Could you check a few things on this drawing? It's one solid part, dimensions in mm from its lowest x, y, z. A direction names the side the tool comes from. Give positions to 0.01 mm unless a question says otherwise; leave off trailing zeros. Write each loop counter-clockwise with the first axis right and the second up, starting at its lowest first coordinate (ties: lowest second). Pieces come first, ordered by that corner, then holes. Notation, with made-up numbers: M 50.25,78 L 96.25,78 A31 ccw 96.25,117 Z; hole C 79.25,9.5 d11. An arc over 180 degrees is marked long. Write each question's results on one line, items separated by ' | '.
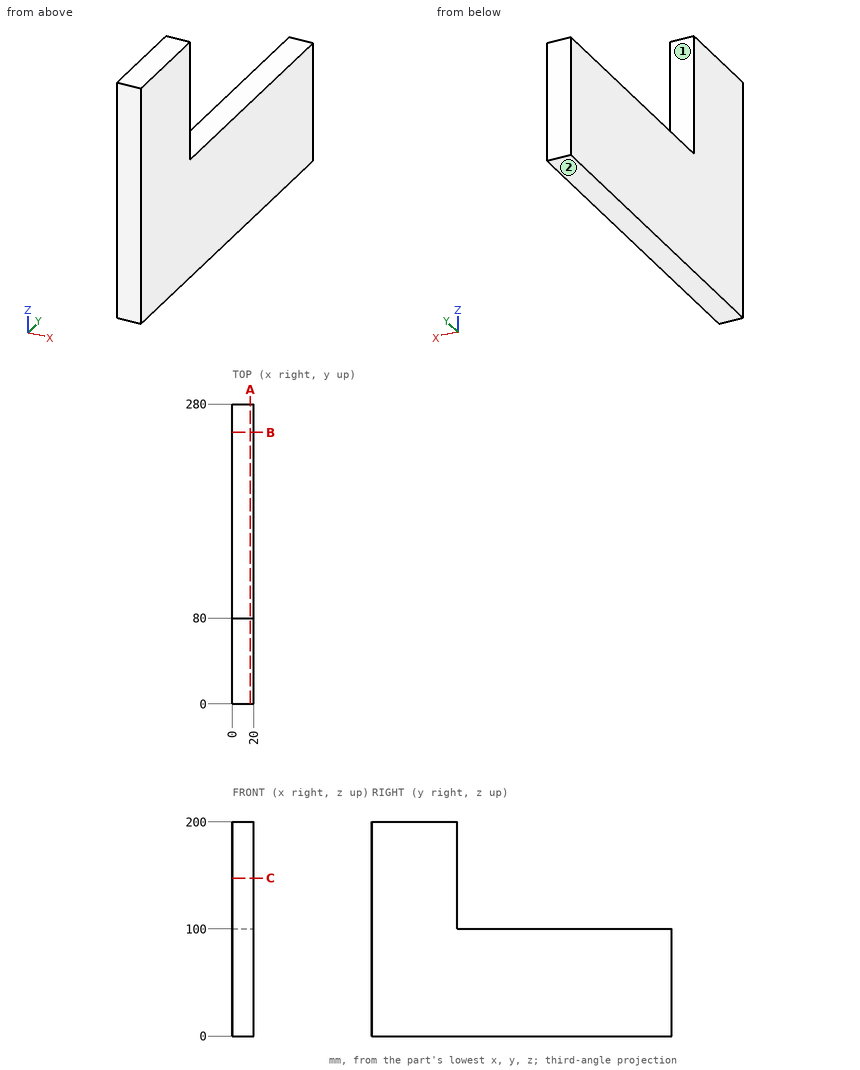
Item 1: I want a section at C-C, the plane z = 147.5. Please give me the cut outline in (x, y).
Geometry says:
outline: M 0,0 L 20,0 L 20,80 L 0,80 Z
Item 2: I want a section at A-A, the plane x = 16.75. Please give me the cut outline in (y, z), and give its area (3 significant figures).
Geometry says:
outline: M 0,0 L 280,0 L 280,100 L 80,100 L 80,200 L 0,200 Z | area: 36,000 mm2
Item 3: I'm going to push flat-ended pins straight in: pin 1 (10 mm diameter, centred on x = 8, z = 157, fed in from +Y); pin 2 (5 mm diameter, centred on x = 10.5, y = 183, fed in from +Z). Where does each tip first touch, or does it pass through?
Geometry says:
pin 1: stops at y = 80 | pin 2: stops at z = 100
Item 4: For the marked faces 1 and 2, which set-ups out of +Z, -Z, +X, -X, +Y, -Y let a thin tool reach every point of the face, with its end or its side?
Geometry says:
face 1: +Z, +X, -X, +Y | face 2: -Z, +X, -X, +Y, -Y
Item 5: If I drill on line 1 (Z direction, x = 6.75, y = 204); line 2 (Y direction, x = 7.75, z = 114), over which ranges is the centre line in solid material (lowest first)? Write a range as from..to.
Geometry says:
line 1: z = 0..100 | line 2: y = 0..80
Item 6: I want a section at B-B, the plane y = 253.5. Please give me the cut outline in (x, z).
Geometry says:
outline: M 0,0 L 20,0 L 20,100 L 0,100 Z
